Geometry check sheet. Reference: the model listing, model coordinates, mm. A direction names the side the tool comes from. Give positions to 0.01 mm unless a question says otherwise; leave off trailing zeros. Write each loop counter-clockwise with the first axis right and the second up, starting at its lowest first coordinate (ties: lowest second). Pieces come first, ordered by that corner, then holes. Notation, with made-up numbers: (70.5, 48) -> (128.5, 48) arc R23 cw to (128.5, 71) -> close; hole circle Ø2 at (-17.5, 63). An arc over 180 degrees is marked (long way). One line per item, written item: value.
from build123d import *

# Parameters (mm, degrees)
SKETCH11_R         = 2
SIZE_4X4_1_DEPTH   = 100
SKETCH12_R         = 2.5
CUT_EXTRUDE1_DEPTH = 10


with BuildPart() as part:
    # Sketch11 → Size 4X4 (1) (new body)
    with BuildSketch(Plane(origin=(0, 0, 0), x_dir=(0, 0, -1), z_dir=(1, 0, 0))):
        with BuildLine():
            Line((-3, 9.2), (-3, 8.8))
            ThreePointArc((-3, 8.8), (-3.234314575, 8.234314575), (-3.8, 8))
            Line((-3.8, 8), (-6.585786438, 8))
            Line((-6.585786438, 8), (-2.820101013, 4.234314575))
            ThreePointArc((-2.820101013, 4.234314575), (-2.560562334, 4.060896374), (-2.254415588, 4))
            Line((-2.254415588, 4), (2.254415588, 4))
            ThreePointArc((2.254415588, 4), (2.560562334, 4.060896374), (2.820101013, 4.234314575))
            Line((2.820101013, 4.234314575), (6.585786438, 8))
            Line((6.585786438, 8), (3.8, 8))
            ThreePointArc((3.8, 8), (3.234314575, 8.234314575), (3, 8.8))
            Line((3, 8.8), (3, 9.2))
            ThreePointArc((3, 9.2), (3.234314575, 9.765685425), (3.8, 10))
            Line((3.8, 10), (9.2, 10))
            ThreePointArc((9.2, 10), (9.765685425, 9.765685425), (10, 9.2))
            Line((10, 9.2), (10, 3.8))
            ThreePointArc((10, 3.8), (9.765685425, 3.234314575), (9.2, 3))
            Line((9.2, 3), (8.8, 3))
            ThreePointArc((8.8, 3), (8.234314575, 3.234314575), (8, 3.8))
            Line((8, 3.8), (8, 6.585786438))
            Line((8, 6.585786438), (4.234314575, 2.820101013))
            ThreePointArc((4.234314575, 2.820101013), (4.060896374, 2.560562334), (4, 2.254415588))
            Line((4, 2.254415588), (4, -2.254415588))
            ThreePointArc((4, -2.254415588), (4.060896374, -2.560562334), (4.234314575, -2.820101013))
            Line((4.234314575, -2.820101013), (8, -6.585786438))
            Line((8, -6.585786438), (8, -3.8))
            ThreePointArc((8, -3.8), (8.234314575, -3.234314575), (8.8, -3))
            Line((8.8, -3), (9.2, -3))
            ThreePointArc((9.2, -3), (9.765685425, -3.234314575), (10, -3.8))
            Line((10, -3.8), (10, -9.2))
            ThreePointArc((10, -9.2), (9.765685425, -9.765685425), (9.2, -10))
            Line((9.2, -10), (3.8, -10))
            ThreePointArc((3.8, -10), (3.234314575, -9.765685425), (3, -9.2))
            Line((3, -9.2), (3, -8.8))
            ThreePointArc((3, -8.8), (3.234314575, -8.234314575), (3.8, -8))
            Line((3.8, -8), (6.585786438, -8))
            Line((6.585786438, -8), (2.820101013, -4.234314575))
            ThreePointArc((2.820101013, -4.234314575), (2.560562334, -4.060896374), (2.254415588, -4))
            Line((2.254415588, -4), (-2.254415588, -4))
            ThreePointArc((-2.254415588, -4), (-2.560562334, -4.060896374), (-2.820101013, -4.234314575))
            Line((-2.820101013, -4.234314575), (-6.585786438, -8))
            Line((-6.585786438, -8), (-3.8, -8))
            ThreePointArc((-3.8, -8), (-3.234314575, -8.234314575), (-3, -8.8))
            Line((-3, -8.8), (-3, -9.2))
            ThreePointArc((-3, -9.2), (-3.234314575, -9.765685425), (-3.8, -10))
            Line((-3.8, -10), (-9.2, -10))
            ThreePointArc((-9.2, -10), (-9.765685425, -9.765685425), (-10, -9.2))
            Line((-10, -9.2), (-10, -3.8))
            ThreePointArc((-10, -3.8), (-9.765685425, -3.234314575), (-9.2, -3))
            Line((-9.2, -3), (-8.8, -3))
            ThreePointArc((-8.8, -3), (-8.234314575, -3.234314575), (-8, -3.8))
            Line((-8, -3.8), (-8, -6.585786438))
            Line((-8, -6.585786438), (-4.234314575, -2.820101013))
            ThreePointArc((-4.234314575, -2.820101013), (-4.060896374, -2.560562334), (-4, -2.254415588))
            Line((-4, -2.254415588), (-4, 2.254415588))
            ThreePointArc((-4, 2.254415588), (-4.060896374, 2.560562334), (-4.234314575, 2.820101013))
            Line((-4.234314575, 2.820101013), (-8, 6.585786438))
            Line((-8, 6.585786438), (-8, 3.8))
            ThreePointArc((-8, 3.8), (-8.234314575, 3.234314575), (-8.8, 3))
            Line((-8.8, 3), (-9.2, 3))
            ThreePointArc((-9.2, 3), (-9.765685425, 3.234314575), (-10, 3.8))
            Line((-10, 3.8), (-10, 9.2))
            ThreePointArc((-10, 9.2), (-9.765685425, 9.765685425), (-9.2, 10))
            Line((-9.2, 10), (-3.8, 10))
            ThreePointArc((-3.8, 10), (-3.234314575, 9.765685425), (-3, 9.2))
        make_face()
        Circle(SKETCH11_R, mode=Mode.SUBTRACT)
    extrude(amount=SIZE_4X4_1_DEPTH)

    # Sketch12 → Cut-Extrude1 (cut)
    with BuildSketch(Plane(origin=(0, 0, -4), x_dir=(-1, 0, 0), z_dir=(0, 0, -1))):
        with Locations(Location((-90, 0, 0), (0, 0, 295.608789007))):
            Circle(SKETCH12_R)
    extrude(amount=-CUT_EXTRUDE1_DEPTH, mode=Mode.SUBTRACT)


solid = part.part
1) Depth check by flat-ended pin: pin 1 Ø6 at (x, z) = (65, 2) entering from +Y; pin 2 Ø3.5 at (x, z) = (33.5, 0.5) entering from +Y; pin 3 Ø3.5 at (x, y) = (32, -0.5) entering from -Z; pin 4 Ø3.5 at (x, z) = (64, -1) entering from -Y. Enter the tip coordinate at first touch or a pass-through.
Verdict:
pin 1: y = 10
pin 2: y = 4
pin 3: z = -4
pin 4: y = -4.17
2) Sectioned sample at A-A on z = 0. Record the cut outline in (x, y), plus the area to 3 significant figures.
Verdict:
outline: (0, -4) -> (100, -4) -> (100, -2) -> (91.5, -2) arc R2.5 cw to (88.5, -2) -> (0, -2) -> close; (0, 2) -> (88.5, 2) arc R2.5 cw to (91.5, 2) -> (100, 2) -> (100, 4) -> (0, 4) -> close
area: 398 mm^2
3) Sectioned sample at B-B on y = 0. Record the cut outline in (x, z).
Verdict:
outline: (0, -4) -> (87.5, -4) -> (87.5, -2) -> (0, -2) -> close; (0, 2) -> (87.5, 2) -> (87.5, 4) -> (0, 4) -> close; (92.5, -4) -> (100, -4) -> (100, -2) -> (92.5, -2) -> close; (92.5, 2) -> (100, 2) -> (100, 4) -> (92.5, 4) -> close
4) Sectioned sample at C-C on y = 5.5. Record the cut outline in (x, z), plus the area to 3 significant figures.
Verdict:
outline: (0, -10) -> (100, -10) -> (100, -8) -> (0, -8) -> close; (0, -6.91) -> (100, -6.91) -> (100, -4.09) -> (0, -4.09) -> close; (0, 4.09) -> (100, 4.09) -> (100, 6.91) -> (0, 6.91) -> close; (0, 8) -> (100, 8) -> (100, 10) -> (0, 10) -> close
area: 966 mm^2
5) Mould release check, pull along Y, two halves, no side actions. Record for faces 1 (the flat face through (49, 7, -10)), 2 (the flat face through (49.3, -4.729, 6.144)), 3 (the flat face through (49, -10, 6)): released by +Y, released by -Y, zero draft, split by the parting line, or undercut.
Verdict:
face 1: zero draft
face 2: undercut
face 3: released by -Y
6) Tool access check on faces 4 (the flat face through (95, 0, 4)), 5 (the flat face through (0, 2.4, -0.1)). Record the directions out of +Z, -Z, +X, -X, +Y, -Y that give a thin tool (end or side, any length) a straight path to the whole face; none if there is none.
Verdict:
face 4: +Z, +X, -X
face 5: +Z, -Z, -X, +Y, -Y
7) Scan lines: probe 1 along Z at (x, y) = (97, 0); probe 2 along Y at (x, z) = (90, -1.75); probe 3 along Y at (x, z) = (59.5, 5.5). Record each from-to range of solid material in increasing order.
Verdict:
probe 1: -4 to -2, 2 to 4
probe 2: -4 to -2.5, 2.5 to 4
probe 3: -10 to -8, -6.91 to -4.09, 4.09 to 6.91, 8 to 10
